Geometry check sheet. Reference: the model listing, model coordinates, mm. Face numbers are marked on the shaded views. A direction names the side the tool comes from. Coordinates: 2 decimals unless noted, no trailing zeros. Write each loop counter-clockwise with the first axis right and the second up, starting at its lowest first coordinate (ties: lowest second). Pieces come first, ordered by that corner, then holes. Notation, with made-up numbers: M -33.5,62.5 L -13.5,62.5 A25 ccw -13.5,87.5 Z; hole C 25,33 d2. An arc over 180 degrees is marked long. Put each result on its own line as item: value. Start each with the question number.
1) Gauge pin test, flat ends, axial feed: pin 1 (3 mm diameter, centred on x = 46.5, y = -51.5, fed in from -Z); pin 2 (14.5 mm diameter, centred on x = 49.5, y = -56, fed in from -Z); pin 3 (6.5 mm diameter, centred on x = 46.3, y = -52.84, fed in from +Z). Record the tip position at first contact, or that the pin passes through.
2) Cross-section at C-C on y = -38.5. Record the cut outline in (x, z), plus the area to 3 significant figures.
3) Cross-section at D-D on x = 55.5. Record the cut outline in (y, z), plus the area to 3 significant figures.
4) Scan lines: line 1 along Y through (x, z) = (53.5, 2.5); line 2 along X through (y, z) = (-57.5, 6.75); line 3 along X through (y, z) = (-62.5, 15). Record each from-to range of solid material in increasing order.
5) Cross-section at A-A on z = 6.25. Record the cut outline in (x, y), plus the area to 3 significant figures.
6) Cross-section at B-B on x = 33. Record the cut outline in (y, z), plus the area to 3 significant figures.
7) Mould release check, pull along Y, two halves, no side actions. Record for the marked faces 1, 2, 3 and 4: released by +Y, released by -Y, zero draft, split by the parting line, or undercut.
8) Set-up check for the marked faces 5, 6 and 7: record each of +Z, -Z, +X, -X, +Y, -Y from which the full face is reachable in a straight line by a thin tool's end or side.
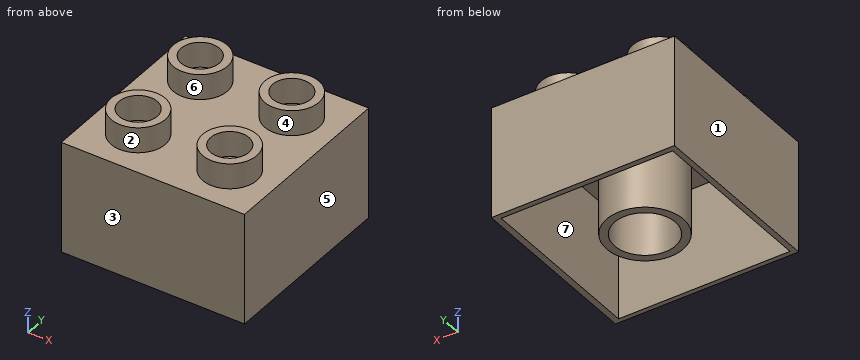
from build123d import *

# Parameters (mm, degrees)
F0_W     = 31.75
F0_H     = 31.75
F1_DEPTH = 19.304
F2_R     = 4.699
F2_R_2   = 3.3147
F3_DEPTH = 4.3942
F4_W     = 29.70818
F4_H     = 30.016836
F5_DEPTH = 17.78
F7_R     = 6.6421
F7_R_2   = 5.2705
F8_DEPTH = 17.653


with BuildPart() as f1:
    # F0 (on Top) → F1 (new body)
    with BuildSketch(Plane.XY):
        with Locations((46.295215, -52.843441)):
            Rectangle(F0_W, F0_H)
    extrude(amount=F1_DEPTH)

    # F2 (on face) → F3 (join)
    with BuildSketch(Plane.XY.offset(19.304)):
        with Locations((38.357715, -44.905941)):
            Circle(F2_R)
        with Locations((38.357715, -44.905941)):
            Circle(F2_R_2, mode=Mode.SUBTRACT)
        with Locations((54.232715, -44.905941)):
            Circle(F2_R)
        with Locations((54.232715, -44.905941)):
            Circle(F2_R_2, mode=Mode.SUBTRACT)
        with Locations((54.232715, -60.780941)):
            Circle(F2_R)
        with Locations((54.232715, -60.780941)):
            Circle(F2_R_2, mode=Mode.SUBTRACT)
        with Locations((38.357715, -60.780941)):
            Circle(F2_R)
        with Locations((38.357715, -60.780941)):
            Circle(F2_R_2, mode=Mode.SUBTRACT)
    extrude(amount=F3_DEPTH)

    # F4 (on face) → F5 (cut)
    with BuildSketch(Plane(origin=(0, 0, 0), x_dir=(1, 0, 0), z_dir=(0, 0, -1))):
        with Locations((46.23173, 52.90393)):
            Rectangle(F4_W, F4_H)
    extrude(amount=-F5_DEPTH, mode=Mode.SUBTRACT)

    # F7 (on face) → F8 (join)
    with BuildSketch(Plane(origin=(0, 0, 17.78), x_dir=(1, 0, 0), z_dir=(0, 0, -1))):
        with Locations((46.295215, 52.843441)):
            Circle(F7_R)
        with Locations((46.295215, 52.843441)):
            Circle(F7_R_2, mode=Mode.SUBTRACT)
    extrude(amount=F8_DEPTH)


solid = f1.part
Answer key:
1. pin 1: stops at z = 17.78
1. pin 2: stops at z = 0.13
1. pin 3: stops at z = 19.3
2. outline: M 30.42,0 L 31.38,0 L 31.38,17.78 L 61.09,17.78 L 61.09,0 L 62.17,0 L 62.17,19.3 L 30.42,19.3 Z
2. area: 84.7 mm²
3. outline: M -68.72,0 L -67.91,0 L -67.91,17.78 L -37.9,17.78 L -37.9,0 L -36.97,0 L -36.97,19.3 L -40.38,19.3 L -40.38,23.7 L -41.84,23.7 L -41.84,19.3 L -47.97,19.3 L -47.97,23.7 L -49.43,23.7 L -49.43,19.3 L -56.26,19.3 L -56.26,23.7 L -57.72,23.7 L -57.72,19.3 L -63.84,19.3 L -63.84,23.7 L -65.31,23.7 L -65.31,19.3 L -68.72,19.3 Z
3. area: 105 mm²
4. line 1: y = -68.72 to -67.91, -37.9 to -36.97
4. line 2: x = 30.42 to 31.38, 41.56 to 43.83, 48.76 to 51.03, 61.09 to 62.17
4. line 3: x = 30.42 to 31.38, 61.09 to 62.17
5. outline: M 30.42,-68.72 L 62.17,-68.72 L 62.17,-36.97 L 30.42,-36.97 Z; C 46.3,-52.84 d13.28; hole M 31.38,-67.91 L 61.09,-67.91 L 61.09,-37.9 L 31.38,-37.9 Z; hole C 46.3,-52.84 d10.54
5. area: 168 mm²
6. outline: M -68.72,0 L -67.91,0 L -67.91,17.78 L -37.9,17.78 L -37.9,0 L -36.97,0 L -36.97,19.3 L -68.72,19.3 Z
6. area: 79.2 mm²
7. face 1: zero draft
7. face 2: undercut
7. face 3: released by -Y
7. face 4: undercut
8. face 5: +Z, -Z, +X, +Y, -Y
8. face 6: +Z
8. face 7: -Z
